Autodesk Inventor part; units mm, degrees
ref_plane "YZ Plane" through (0, 0, 0) normal (1, 0, 0) x (0, 1, 0)
ref_plane "XZ Plane" through (0, 0, 0) normal (0, 1, 0) x (-1, 0, 0)
ref_plane "XY Plane" through (0, 0, 0) normal (0, 0, 1) x (1, 0, 0)
sketch "Sketch1" plane through (0, 0, 0) normal (0, 1, 0) x (-1, 0, 0)
  circle A0 centre (0, 0) radius 6.3
  dimension "d0" = 12.6
extrude "Extrusion1" add sketch "Sketch1" along normal mid plane 127
sketch "Sketch2" plane through (0, 0, 0) normal (1, 0, 0) x (0, 1, 0)
  line L0 (63.5, -6.3) -> (63.5, 6.3)
  line L1 (-63.5, -6.3) -> (63.5, -6.3)
  line L2 (63.5, 6.3) -> (51.87, 6.3)
  line L3 (51.87, 6.3) -> (51.87, -6.3)
  line L4 (51.87, -6.3) -> (63.5, -6.3)
  line L5 (63.5, -6.3) -> (63.5, 6.3)
  line L6 (63.5, 0) -> (58.5, 0)
  circle A0 centre (58.5, 0) radius 3
  point P0 (0, 0)
  dimension "d3" = 11.63
  dimension "d7" = 5
  dimension "d8" = 6
sketch "Sketch3" plane through (0, 63.5, 0) normal (0, 1, 0) x (1, 0, 0)
  circle A0 centre (0, 0) radius 6.3
  line L0 (2, -5.9741) -> (-2, -5.9741)
  line L1 (-2, -5.9741) -> (-2, 5.9741)
  line L2 (-2, 5.9741) -> (2, 5.9741)
  line L3 (2, 5.9741) -> (2, -5.9741)
  line L4 (2, -5.9741) -> (-2, 5.9741) construction
  line L5 (-2, -5.9741) -> (2, 5.9741) construction
  dimension "d4" = 4
extrude "Extrusion2" cut sketch "Sketch3" against normal blind 11.63 contours A0 L3 | L1 A0
extrude "Extrusion3" cut sketch "Sketch2" against normal mid plane 11.63 contours A0
sketch "Sketch4" plane through (0, -63.5, 0) normal (0, -1, 0) x (1, 0, 0)
  circle A0 centre (0, 0) radius 7.25
  dimension "d11" = 14.5
extrude "Extrusion4" add sketch "Sketch4" against normal blind 10
properties part number "SP6V1 Vastago Freno" material "Stainless Steel"
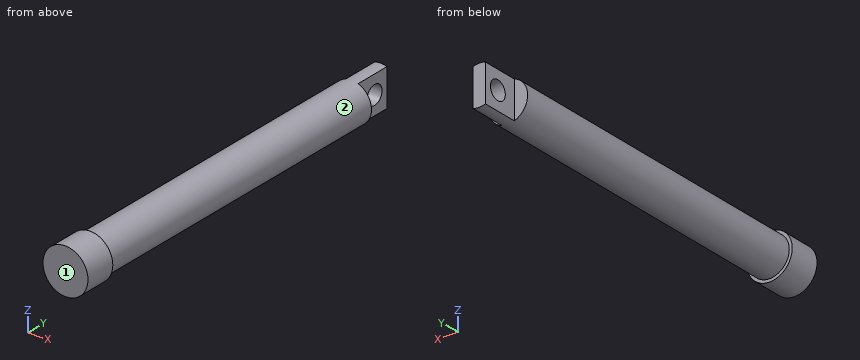
Part model, mm, in its own coordinate system. Face numbers are marked on the shaded views. A direction names the side the tool comes from. Round coordinates to 2 decimals unless told otherwise and drop trailing zeros. Loops run counter-clockwise (first coordinate to the right, second up) from the corner with the lowest first, then second, coordinate; pieces in that order, holes last. Notation, with made-up numbers: (12.5, -16) -> (40.5, -16) arc R21 ccw to (40.5, 14) -> close; hole circle Ø2 at (-15.5, -33). An arc over 180 degrees is marked (long way). Use CSV: the item, a comma, the result in double quotes. Start each with the question number.
1) Cut at D-D, the plane y = -32. Write the cut outline in (x, z).
2) Drop flat-ended pins along their axis: P1, Ø4, axis at x = 4.5, y = -34, coming from the +Z side; P2, Ø5, axis at x = -1, y = 17.5, coming from the -Z side; P3, Ø5, axis at y = 18.5, z = 2.5, coming from the +X side. Give the stop position or say it passes through.
3) Cut at B-B, the plane y = 58.5. Write the cut outline in (x, z).
4) Cut at C-C, the plane z = 0. Write the cut outline in (x, y), plus the area to 3 significant figures.
5) Wall check: L1, parallel to Z at x = -0.3, y = 58.5; L2, parallel to Z at x = 2, y = -8; L3, parallel to Y at x = -5.5, z = -3.75. Give the ranges that are in metal, low to high. Write a range as [from, to].
6) Cut at A-A, the plane x = 0. Write the cut outline in (y, z), plus the area to 3 significant figures.
7) Which spindle directions (+Z, -Z, +X, -X, +Y, -Y) get a long thin tool onto all of the face, cutting with end or side? Do the marked faces 1 and 2. Say none if no direction does.
Determined:
1,outline,"circle Ø12.6 at (0, 0)"
2,P1,"stops at z = 5.78"
2,P2,"stops at z = -6.3"
2,P3,"stops at x = 6.3"
3,outline,"(-2, -5.97) arc R6.3 ccw to (2, -5.97) -> (2, -3) -> (-2, -3) -> close; (-2, 3) -> (2, 3) -> (2, 5.97) arc R6.3 ccw to (-2, 5.97) -> close"
4,outline,"(-7.25, -63.5) -> (7.25, -63.5) -> (7.25, -53.5) -> (6.3, -53.5) -> (6.3, 51.87) -> (2, 51.87) -> (2, 55.5) -> (-2, 55.5) -> (-2, 51.87) -> (-6.3, 51.87) -> (-6.3, -53.5) -> (-7.25, -53.5) -> close; (-2, 61.5) -> (2, 61.5) -> (2, 63.5) -> (-2, 63.5) -> close"
4,area,"1,500 mm2"
5,L1,"z = [-6.29, -3], [3, 6.29]"
5,L2,"z = [-5.97, 5.97]"
5,L3,"y = [-63.5, -53.5]"
6,outline,"(-63.5, -7.25) -> (-53.5, -7.25) -> (-53.5, -6.3) -> (63.5, -6.3) -> (63.5, 6.3) -> (-53.5, 6.3) -> (-53.5, 7.25) -> (-63.5, 7.25) -> close; hole circle Ø6 at (58.5, 0)"
6,area,"1,590 mm2"
7,face 1,"+Z, -Z, +X, -X, -Y"
7,face 2,"+Y"
